```python
from build123d import *

# Parameters (mm, degrees)
EXTRUDE1_DEPTH = 15
FILLET1_R      = 0.5


with BuildPart() as part:
    # Sketch2 → Extrude1 (new, symmetric)
    with BuildSketch(Plane.XY):
        with BuildLine():
            Line((-2.593415235, 0.045802636), (-2.538323026, -0.401884053))
            ThreePointArc((-2.538323026, -0.401884053), (0.045183933, -2.569603849), (2.550988586, -0.312512721))
            Line((2.550988586, -0.312512721), (2.594832844, 0.045372131))
            ThreePointArc((2.594832844, 0.045372131), (2.899006177, 0.58055361), (3.493240793, 0.741257846))
            Line((3.493240793, 0.741257846), (3.666713736, 2.059896211))
            Line((3.666713736, 2.059896211), (0.028937175, 2.059896211))
            Line((0.028937175, 2.059896211), (0.028937175, 2.258712577))
            Line((0.028937175, 2.258712577), (0.028937175, 2.299985842))
            Line((0.028937175, 2.299985842), (-0.027466707, 2.299985842))
            Line((-0.027466707, 2.299985842), (-0.027466707, 2.258712577))
            Line((-0.027466707, 2.258712577), (-0.027466707, 2.059896211))
            Line((-0.027466707, 2.059896211), (-3.665243268, 2.059896211))
            Line((-3.665243268, 2.059896211), (-3.491770325, 0.741257846))
            ThreePointArc((-3.491770325, 0.741257846), (-2.897707177, 0.580686389), (-2.593415235, 0.045802636))
        make_face()
    extrude(amount=EXTRUDE1_DEPTH, both=True)

    # Fillet1
    fillet1_edges = [part.edges().sort_by_distance(p)[0] for p in [
        (-3.491770325, 0.741257846, 0),
        (3.493240793, 0.741257846, 0),
    ]]
    fillet(fillet1_edges, radius=FILLET1_R)


solid = part.part
```
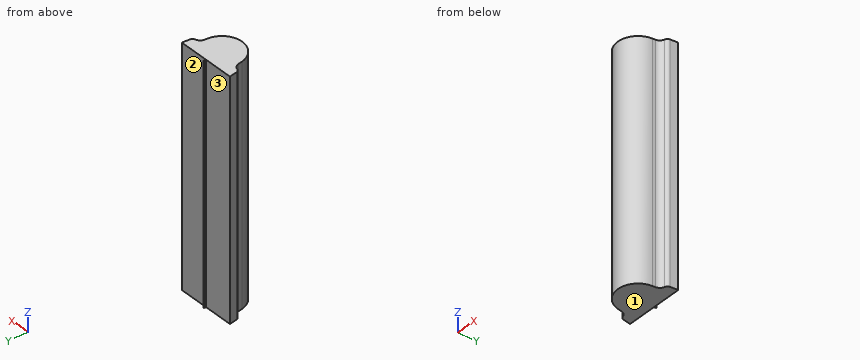
Could you check a few things on this model? Use its own coordinates, in mm. Face numbers are marked on the shaded views. A direction names the side the tool comes from. Round coordinates to 2 decimals unless told otherwise and drop trailing zeros. Loops run counter-clockwise (first coordinate to the right, second up) from the corner with the lowest first, then second, coordinate; pieces in that order, holes last.
Q1. Please list where these lines run through material, in increasing order: L1, parallel to Y at x = -0.75, z = -0.5; L2, parallel to X at y = -1.3, z = 2.75; L3, parallel to X at y = 1.2, z = 6.75.
Q2. I want a section at A-A (z = 2). Write out the boundary of the cut face in (x, y).
Q3. For P1, Ø3, axis at x = 2.5, z = 5, coming from the +Y side, with a flat end and sliding along its axis, tell me the tip position at first contact or that it passes through.
Q4. On a 3-axis mill with a long thin cutter (end or side, diameter ignored), from which of +Z, -Z, +X, -X, +Y, -Y can I reach the whole of each face in a straight line? I mean the marked faces 1, 2 and 3. Say none if no direction works.
Q5. I want a section at B-B (y = -1.9). Write out the boundary of the cut face in (x, z).
Q6. I want a section at C-C (x = -0.75). Write out the boundary of the cut face in (y, z).
Answer below:
1. L1: y = -2.46 to 2.06
1. L2: x = -2.22 to 2.22
1. L3: x = -3.55 to 3.55
2. outline: (-3.67, 2.06) - (-3.54, 1.14) arc R0.5 ccw to (-3.18, 0.72) arc R0.8 cw to (-2.59, 0.05) - (-2.54, -0.4) arc R2.57 ccw to (2.55, -0.31) - (2.59, 0.05) arc R0.8 cw to (3.18, 0.72) arc R0.5 ccw to (3.55, 1.14) - (3.67, 2.06) - (0.03, 2.06) - (0.03, 2.3) - (-0.03, 2.3) - (-0.03, 2.06) - close
3. P1: stops at y = 2.06
4. face 1: -Z, +X, -X, +Y, -Y
4. face 2: +Z, -Z, +X, +Y
4. face 3: +Z, -Z, -X, +Y
5. outline: (-1.73, -15) - (1.73, -15) - (1.73, 15) - (-1.73, 15) - close
6. outline: (-2.46, -15) - (2.06, -15) - (2.06, 15) - (-2.46, 15) - close
